Input: part model. Units: mm. Frame: model coordinates. Face numbers are marked on the shaded views. A direction names the side the tool comes from. Give positions to 0.01 mm unless a question says otherwise; leave off trailing zeros. Loops run counter-clockwise (first coordinate to the right, second up) from the corner with the lowest first, then second, coordinate; pieces in that order, holes last. Notation, with made-up numbers: (31, -26) -> (62, -26) arc R21 cw to (62, -14) -> close; hole circle Ø9 at (-2.5, 63.25). An arc over 180 degrees is marked (long way). Answer in a Markdown table with one row per item. Add a question column.
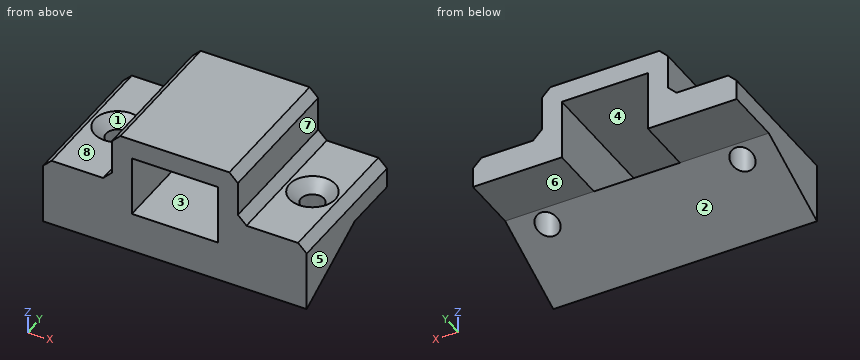
```python
from build123d import *

# Parameters (mm, degrees)
F1_DEPTH        = 11
F2_W            = 15
F2_H            = 10.5
F3_DEPTH        = 25.001
F5_DEPTH        = 12
F7_DEPTH        = 12
F8_SIZE         = 1.5
F10_D           = 4
F10_CSINK_D     = 8
F10_CSINK_ANGLE = 90


with BuildPart() as f1:
    # F0 (on Right) → F1 (new body, symmetric)
    with BuildSketch(Plane.YZ):
        Polygon((-15, -7), (0, 0), (10, 0), (10, 14), (-15, 14), align=None)
    extrude(amount=F1_DEPTH, both=True)

    # F2 (on face) → F3 (cut, through all)
    with BuildSketch(Plane(origin=(0, 10, 0), x_dir=(-1, 0, 0), z_dir=(0, 1, 0))):
        with Locations((0, 5.25)):
            Rectangle(F2_W, F2_H)
    extrude(amount=-F3_DEPTH, mode=Mode.SUBTRACT)

    # F4 (on face) → F5 (join)
    with BuildSketch(Plane(origin=(-11, 0, 0), x_dir=(0, -1, 0), z_dir=(-1, 0, 0))):
        Polygon((15, 5), (-10, 5), (-10, 0), (0, 0), (15, -7), align=None)
    extrude(amount=F5_DEPTH)

    # F6 (on face) → F7 (join)
    with BuildSketch(Plane.YZ.offset(11)):
        Polygon((10, 0), (10, 5), (-15, 5), (-15, -7), (0, 0), align=None)
    extrude(amount=F7_DEPTH)

    # F8
    f8_edges = [f1.edges().sort_by_distance(p)[0] for p in [
        (11, -2.5, 5),
        (11, -2.5, 14),
        (-11, -2.5, 14),
        (-11, -2.5, 5),
        (23, -2.5, 5),
        (-23, -2.5, 5),
    ]]
    chamfer(f8_edges, length=F8_SIZE)

    # F10 (through all)
    with Locations(Plane.XY.offset(5)):
        with Locations((-17, -2.5), (17, -2.5)):
            CounterSinkHole(F10_D / 2, F10_CSINK_D / 2, counter_sink_angle=F10_CSINK_ANGLE)


solid = f1.part
```
1) Section B-B on y = -2.5. State how many separate pieces and enclosed holes the cut face has, and give its area (3 significant figures).
2) Section A-A on z = 5.5. Output: boundary loops of the cut face in (x, y).
3) Reachability of the marked faces 4, 5, 6, 7 and 8 from +Z, -Z, +X, -X, +Y, -Y: full face, straight path, thin tool, end or side. Return the list, or none.
4) Material intervals for line 1 along X through (y, z) = (-2.5, -0.35); line 2 along X through (y, z) = (-2.5, 0.55); line 3 along X through (y, z) = (-2, 2), sorted ascending.
5) Section D-D on y = -9.25. Output: boundary loops of the cut face in (x, z).
6) Pin query (flat end, axial travel): pin 1 (5 mm diameter, centred on x = -17, y = -2.5, fed in from -Z); pin 2 (1.8 mm diameter, centred on y = -0.5, z = 10.5, fed in from -X); pin 3 (12 mm diameter, centred on x = -12.5, y = -7.5, fed in from -Z). Return the tip coordinate at first contact, or that it passes through.
7) Pull-direction query (Y, two-part tool) for the marked faces 1, 2 and 3; classes: +Y half, -Y half, draft (parallel to the pull), parting line (faces both ways), or undercut.
8) Section C-C on x = 17. Output: boundary loops of the cut face in (y, z).
Working result:
| question | item | result |
|---|---|---|
| 1 | separate pieces | 3 |
| 1 | enclosed holes | 1 |
| 1 | area | 265 mm2 |
| 2 | outline | (-12, -15) -> (-7.5, -15) -> (-7.5, 10) -> (-12, 10) -> close; (7.5, -15) -> (12, -15) -> (12, 10) -> (7.5, 10) -> close |
| 3 | face 4 | +Y, -Y |
| 3 | face 5 | +Z, -Z, +X, +Y, -Y |
| 3 | face 6 | -Z, +X, -X, +Y |
| 3 | face 7 | +Z, +X, +Y, -Y |
| 3 | face 8 | +Z, -X, +Y, -Y |
| 4 | line 1 | x = -23 to -19, -15 to 15, 19 to 23 |
| 4 | line 2 | x = -23 to -19, -15 to -7.5, 7.5 to 15, 19 to 23 |
| 4 | line 3 | x = -23 to -18.94, -15.06 to -7.5, 7.5 to 15.06, 18.94 to 23 |
| 5 | outline | (-23, -4.32) -> (23, -4.32) -> (23, 3.5) -> (21.5, 5) -> (12.5, 5) -> (11, 6.5) -> (11, 12.5) -> (9.5, 14) -> (-9.5, 14) -> (-11, 12.5) -> (-11, 6.5) -> (-12.5, 5) -> (-21.5, 5) -> (-23, 3.5) -> close; hole (-7.5, 0) -> (7.5, 0) -> (7.5, 10.5) -> (-7.5, 10.5) -> close |
| 6 | pin 1 | stops at z = -2.33 |
| 6 | pin 2 | stops at x = -11 |
| 6 | pin 3 | stops at z = -6.3 |
| 7 | face 1 | undercut |
| 7 | face 2 | +Y half |
| 7 | face 3 | draft |
| 8 | outline | (-15, -7) -> (-4.5, -2.1) -> (-4.5, 3) -> (-6.5, 5) -> (-15, 5) -> close; (-0.5, -0.23) -> (0, 0) -> (10, 0) -> (10, 5) -> (1.5, 5) -> (-0.5, 3) -> close |
